CAD build for the part. Positions are in the model's coordinates, mm. Face numbers are marked on the shaded views. A direction names the side the tool comes from. Round coordinates to 2 decimals unless told otherwise and drop trailing zeros. Loops run counter-clockwise (first coordinate to the right, second up) from the corner with the lowest first, then second, coordinate; pieces in that order, holes last.
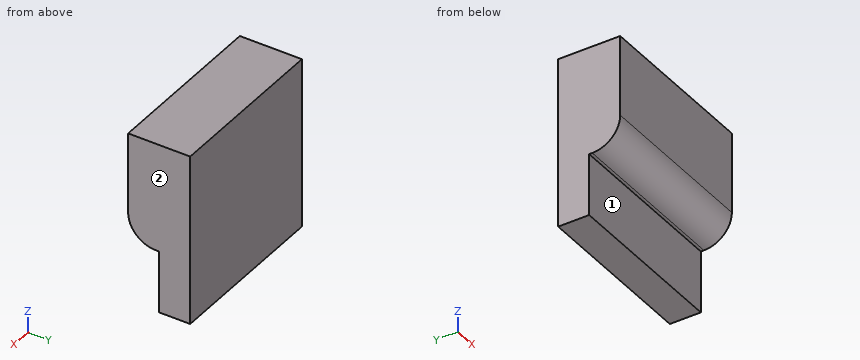
from build123d import *

# Parameters (mm, degrees)
BOX023_W     = 5.5
BOX023_H     = 1
BOX023_DEPTH = 2
BOX022_W     = 5.5
BOX022_H     = 2
BOX022_DEPTH = 5.5
FILLET005_R  = 0.9


with BuildPart() as button_1_cut003:
    # Box023 → Box023 (new body)
    with BuildSketch(Plane(origin=(5, 24, -15), x_dir=(1, 0, 0), z_dir=(0, 0, 1))):
        with Locations((2.75, 0.5)):
            Rectangle(BOX023_W, BOX023_H)
    extrude(amount=BOX023_DEPTH)


with BuildPart() as fillet005:
    # Box022 → Box022 (new body)
    with BuildSketch(Plane(origin=(5, 24, -15), x_dir=(1, 0, 0), z_dir=(0, 0, 1))):
        with Locations((2.75, 1)):
            Rectangle(BOX022_W, BOX022_H)
    extrude(amount=BOX022_DEPTH)

    # Cut003: cut Button 1 Cut003
    add(button_1_cut003.part, mode=Mode.SUBTRACT)

    # Fillet005
    fillet005_edges = [fillet005.edges().sort_by_distance(p)[0] for p in [
        (7.75, 24, -13),
    ]]
    fillet(fillet005_edges, radius=FILLET005_R)


with BuildPart() as fillet005_1:
    # Fillet005 placement: moved
    add(fillet005.part.moved(Location((-21, 0, 0))))


solid = fillet005_1.part
Item 1: Cut at B-B (z = -13.85). List the corners of the cut face in (x, y).
Verdict:
outline: (-16, 25) - (-10.5, 25) - (-10.5, 26) - (-16, 26) - close
Item 2: Cut at A-A (x = -15.4). List the corners of the cut face in (y, z).
Verdict:
outline: (24, -12.1) arc R0.9 ccw to (24.9, -13) - (25, -13) - (25, -15) - (26, -15) - (26, -9.5) - (24, -9.5) - close
Item 3: 3-axis set-ups, long thin cutter, end or side, ignore diameter. For the marked faces 1 and 2: which of +Z, -Z, +X, -X, +Y, -Y reach the whole face in a straight line?
Verdict:
face 1: -Z, +X, -X, -Y
face 2: +Z, -Z, +X, +Y, -Y
Item 4: Cut at C-C (y = 24.45). List the corners of the cut face in (x, z), plus the area to 3 significant figures.
Verdict:
outline: (-16, -12.88) - (-10.5, -12.88) - (-10.5, -9.5) - (-16, -9.5) - close
area: 18.6 mm2
Item 5: Wall check: L1, parallel to Y at x = -12.6, z = -13.45; L2, parallel to Z at x = -14.7, y = 24.3; L3, parallel to Y at x = -11.45, z = -12.75. Give the ranges that are in metal, low to high.
Verdict:
L1: y = 25 to 26
L2: z = -12.77 to -9.5
L3: y = 24.28 to 26
Item 6: Flat gauge pin, fed straight in: P1, Ø2, axis at x = -14.5, z = -14.5, coming from the -Y side. Where does the tip first touch, or does it go through?
Verdict:
P1: stops at y = 25
